For this review, use the dimensioned drawing (mm, ordinates from the lowest corner) and the shaded views. A direction names the side the tool comes from. Coordinates: 2 decimals unless noted, no trailing zeros. Loops run counter-clockwise (first coordinate to the right, second up) from the corner with the lowest first, then second, coordinate; pieces in that order, holes last.
1. Take a section at A-A, the plane y = 9.25. State the section outline as (x, z) points, then the cut area to 3 significant figures.
2. Clearance check with flat-ended pins moving along their axes: P1, Ø3, axis at x = 11.5, y = 8, coming from the -Z side; P2, Ø3.5, axis at x = 96, z = 15, coming from the +Y side. State where each tip first meets the part, or that it passes through.
3. Machinability: for the marked faces 1 and 2, which of the approach directions +Z, -Z, +X, -X, +Y, -Y give a long, thin tool a straight path to every point of the face, cutting with its end or side? Answer none if there is none.
4. Take a section at B-B, the plane x = 5. State the section outline as (y, z) points (3 decimals).
5. To check wall thickness, follow probe 1 along X at (y, z) = (19.85, 15) (3 decimals); probe 2 along Z at (x, y) = (96, 0.65) (3 decimals); probe 3 along Z at (x, y) = (15.5, 5.75). State the ranges of each line that lie inside material, in increasing order.
6. Mouldability with a two-part tool opening along Z and no side actions: class the marked faces 3, 4 and 5 as pulls with the +Z half, pulls with the -Z half, needs draft (parallel to the pull), parting line crosses it, or undercut.
7. Take a section at D-D, the plane x = 71.5. State the section outline as (y, z) points, then the cut area to 3 significant figures.
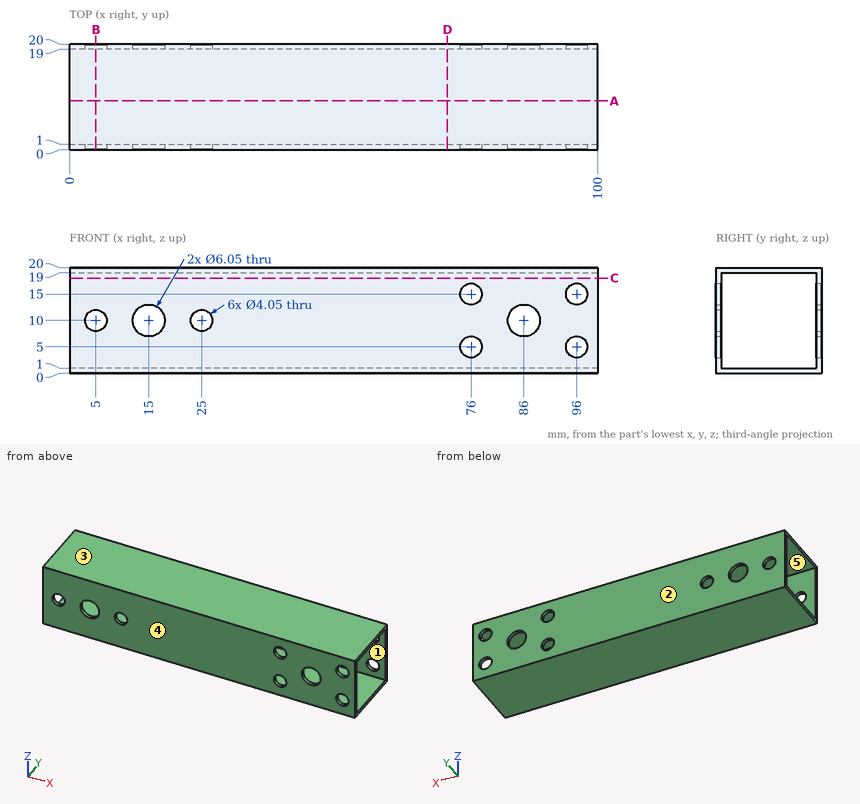
Results list:
1. outline: (0, 0) - (100, 0) - (100, 1) - (0, 1) - close; (0, 19) - (100, 19) - (100, 20) - (0, 20) - close
1. area: 200 mm2
2. P1: stops at z = 0
2. P2: passes through
3. face 1: +X, -X
3. face 2: +Z, -Z, +X, -X, +Y
4. outline: (0, 0) - (20, 0) - (20, 7.975) - (19, 7.975) - (19, 1) - (1, 1) - (1, 7.975) - (0, 7.975) - close; (0, 12.025) - (1, 12.025) - (1, 19) - (19, 19) - (19, 12.025) - (20, 12.025) - (20, 20) - (0, 20) - close
5. probe 1: x = 0 to 73.975, 78.025 to 93.975, 98.025 to 100
5. probe 2: z = 0 to 2.975, 7.025 to 12.975, 17.025 to 20
5. probe 3: z = 0 to 1, 19 to 20
6. face 3: pulls with the +Z half
6. face 4: needs draft
6. face 5: undercut
7. outline: (0, 0) - (20, 0) - (20, 20) - (0, 20) - close; hole (1, 1) - (19, 1) - (19, 19) - (1, 19) - close
7. area: 76.0 mm2
